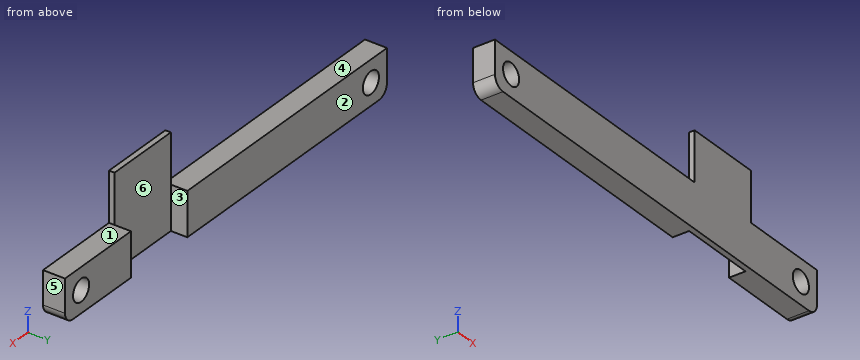
from build123d import *

# Parameters (mm, degrees)
EXTRUDE_1_DEPTH     = 12
CUT_EXTRUDE_1_DEPTH = 12
SKETCH_3_R          = 2
CUT_EXTRUDE_2_DEPTH = 12
CUT_EXTRUDE_3_DEPTH = 1
SKETCH_5_W          = 80
SKETCH_5_H          = 4
CUT_EXTRUDE_4_DEPTH = 20
EXTRUDE_2_DEPTH     = 1
SKETCH_7_W          = 0.2
SKETCH_7_H          = 8
CUT_EXTRUDE_5_DEPTH = 1
SKETCH_8_R          = 2
EXTRUDE_3_DEPTH     = 4
SKETCH_9_W          = 80
SKETCH_9_H          = 8
CUT_EXTRUDE_6_DEPTH = 10
SKETCH_10_W         = 14
SKETCH_10_H         = 8
CUT_EXTRUDE_7_DEPTH = 2
SKETCH_11_W         = 14
SKETCH_11_H         = 9
EXTRUDE_4_DEPTH     = 2
SKETCH_12_W         = 14
SKETCH_12_H         = 1
CUT_EXTRUDE_8_DEPTH = 20


with BuildPart() as part:
    # 草图1 → 凸台-拉伸1 (new body)
    with BuildSketch(Plane(origin=(0, 0, 0), x_dir=(1, 0, 0), z_dir=(0, 1, 0))):
        Polygon((-40, -6), (0, -6), (40, -6), (40, 0), (40, 6), (0, 6), (-36, 6), (-40, 6), align=None)
    extrude(amount=EXTRUDE_1_DEPTH)

    # 草图2 → 切除-拉伸1 (cut)
    with BuildSketch(Plane.XY.offset(6)):
        Polygon((-28, 0), (0, 0), (28, 0), (28, 4), (28, 8), (-28, 8), (-28, 4), align=None)
        Polygon((-40, 4), (-32, 4), (-32, 8), (-32, 12), (-40, 12), align=None)
        Polygon((32, 8), (32, 4), (40, 4), (40, 12), (32, 12), align=None)
    extrude(amount=-CUT_EXTRUDE_1_DEPTH, mode=Mode.SUBTRACT)

    # 草图3 → 切除-拉伸2 (cut)
    with BuildSketch(Plane(origin=(0, 12, 0), x_dir=(1, 0, 0), z_dir=(0, 1, 0))):
        with BuildLine():
            Line((-40, 6), (-40, 4))
            ThreePointArc((-40, 4), (-39.414213562, 5.414213562), (-38, 6))
            Line((-38, 6), (-40, 6))
        make_face()
        with Locations(Location((-36, 2, 0), (0, 0, 270))):
            Circle(SKETCH_3_R)
        with BuildLine():
            ThreePointArc((40, 4), (39.414213562, 5.414213562), (38, 6))
            Line((38, 6), (40, 6))
            Line((40, 6), (40, 4))
        make_face()
        with Locations(Location((36, 2, 0), (0, 0, 270))):
            Circle(SKETCH_3_R)
    extrude(amount=-CUT_EXTRUDE_2_DEPTH, mode=Mode.SUBTRACT)

    # 草图4 → 切除-拉伸3 (cut)
    with BuildSketch(Plane(origin=(0, 12, 0), x_dir=(1, 0, 0), z_dir=(0, 1, 0))):
        Polygon((-21.1, 0), (-21.1, 6), (-16.6, 6), (-12.1, 6), (12.08, 6), (16.6, 6), (21.12, 6), (21.12, -1), (21.12, -6), (16.6, -6), (12.08, -6), (12.08, -1), (12.08, 0), (-12.1, 0), (-12.1, -6), (-16.6, -6), (-21.1, -6), align=None)
    extrude(amount=-CUT_EXTRUDE_3_DEPTH, mode=Mode.SUBTRACT)

    # 草图5 → 切除-拉伸4 (cut)
    with BuildSketch(Plane(origin=(0, 12, 0), x_dir=(1, 0, 0), z_dir=(0, 1, 0))):
        with Locations((0, -4)):
            Rectangle(SKETCH_5_W, SKETCH_5_H)
    extrude(amount=-CUT_EXTRUDE_4_DEPTH, mode=Mode.SUBTRACT)

    # 草图6 → 凸台-拉伸2 (add)
    with BuildSketch(Plane(origin=(0, 12, 0), x_dir=(1, 0, 0), z_dir=(0, 1, 0))):
        Polygon((12.08, 0), (12.08, 6), (-21.1, 6), (-21.1, -2), (-12.1, -2), (-12.1, 0), align=None)
    extrude(amount=-EXTRUDE_2_DEPTH)

    # 草图7 → 切除-拉伸5 (cut)
    with BuildSketch(Plane(origin=(0, 12, 0), x_dir=(1, 0, 0), z_dir=(0, 1, 0))):
        with Locations((21.22, 2)):
            Rectangle(SKETCH_7_W, SKETCH_7_H)
        with Locations((11.98, 2)):
            Rectangle(SKETCH_7_W, SKETCH_7_H)
    extrude(amount=-CUT_EXTRUDE_5_DEPTH, mode=Mode.SUBTRACT)

    # 草图8 → 凸台-拉伸3 (add)
    # profile 1 of 2: a face of its own
    with BuildSketch(Plane(origin=(0, 12, 0), x_dir=(1, 0, 0), z_dir=(0, 1, 0))):
        with BuildLine():
            Line((-32, -2), (-40, -2))
            Line((-40, -2), (-40, 4))
            ThreePointArc((-40, 4), (-39.414213562, 5.414213562), (-38, 6))
            Line((-38, 6), (-32, 6))
            Line((-32, 6), (-32, -2))
        make_face()
        with Locations(Location((-36, 2, 0), (0, 0, 270))):
            Circle(SKETCH_8_R, mode=Mode.SUBTRACT)
    # profile 2 of 2: a face of its own
    with BuildSketch(Plane(origin=(0, 12, 0), x_dir=(1, 0, 0), z_dir=(0, 1, 0))):
        with BuildLine():
            Line((32, -2), (32, 6))
            Line((32, 6), (38, 6))
            ThreePointArc((38, 6), (39.414213562, 5.414213562), (40, 4))
            Line((40, 4), (40, -2))
            Line((40, -2), (32, -2))
        make_face()
        with Locations(Location((36, 2, 0), (0, 0, 270))):
            Circle(SKETCH_8_R, mode=Mode.SUBTRACT)
    extrude(amount=-EXTRUDE_3_DEPTH)

    # 草图9 → 切除-拉伸6 (cut)
    with BuildSketch(Plane.XY.offset(2)):
        with Locations((0, 4)):
            Rectangle(SKETCH_9_W, SKETCH_9_H)
    extrude(amount=-CUT_EXTRUDE_6_DEPTH, mode=Mode.SUBTRACT)

    # 草图10 → 切除-拉伸7 (cut)
    with BuildSketch(Plane(origin=(0, 12, 0), x_dir=(1, 0, 0), z_dir=(0, 1, 0))):
        with Locations((16.6, 2)):
            Rectangle(SKETCH_10_W, SKETCH_10_H)
    extrude(amount=-CUT_EXTRUDE_7_DEPTH, mode=Mode.SUBTRACT)

    # 草图11 → 凸台-拉伸4 (add)
    with BuildSketch(Plane(origin=(0, 10, 0), x_dir=(1, 0, 0), z_dir=(0, 1, 0))):
        with Locations((16.6, -6.5)):
            Rectangle(SKETCH_11_W, SKETCH_11_H)
    extrude(amount=-EXTRUDE_4_DEPTH)

    # 草图12 → 切除-拉伸8 (cut)
    with BuildSketch(Plane(origin=(0, 0, -6), x_dir=(-1, 0, 0), z_dir=(0, 0, -1))):
        with Locations((-16.6, 9.5)):
            Rectangle(SKETCH_12_W, SKETCH_12_H)
    extrude(amount=-CUT_EXTRUDE_8_DEPTH, mode=Mode.SUBTRACT)


solid = part.part
For this review, take the finished solid that the model builds, in its own axes (mm). Face numbers are marked on the shaded views. A direction names the side the tool comes from. Give positions to 0.01 mm unless a question says otherwise; leave off trailing zeros. Loops run counter-clockwise (first coordinate to the right, second up) from the corner with the lowest first, then second, coordinate; pieces in that order, holes last.
Item 1: Draft analysis for pull direction X (two halves, no side actions). For the marked faces 4, 5 and 6, state which applies: +X half, -X half, draft (parallel to the pull), parting line (faces both ways), or undercut.
Item 2: Tool access review of the marked faces 1, 2 and 3: name each direction out of +Z, -Z, +X, -X, +Y, -Y from which nothing blocks a thin tool from reaching the whole face with its end or side.
Item 3: Take a section at C-C, the plane z = 1.25. State the section outline as (x, y) points.
Item 4: Take a section at A-A, the plane x = 36. State the section outline as (y, z) points.
Item 5: For line 1 along X through (y, z) = (11.15, 0.25); line 2 along Z through (x, y) = (-3, 11.45); line 3 along Z through (x, y) = (37, 10.85), list the stretches that pass through material, from the lowest coordinate up.
Item 6: Insertion check: pin 1 (1.1 mm diameter, centred on y = 8.5, z = 7.5, fed in from -X); pin 2 (2 mm diameter, centred on x = -8.5, y = 10, fed in from +Z); pin 3 (1.1 mm diameter, centred on y = 8.5, z = 8, fed in from +X). Each pin has a flat end and moves straight along its axis. Give the tip position at first contact, or say it passes through.
Item 7: Take a section at D-D, the plane x = 8. State the section outline as (y, z) points.
Item 8: Take a section at B-B, the plane z = -2. State the section outline as (x, y) points.
Calculated:
1. face 4: draft
1. face 5: +X half
1. face 6: undercut
2. face 1: +Z, +X, +Y, -Y
2. face 2: +Z, -Z, +X, -X, +Y
2. face 3: +Z, -Z, +Y
3. outline: (-40, 8) - (40, 8) - (40, 12) - (23.6, 12) - (23.6, 9) - (9.6, 9) - (9.6, 12) - (-40, 12) - close
4. outline: (8, -6) - (12, -6) - (12, -4) - (8, -4) - close; (8, 0) - (12, 0) - (12, 2) - (8, 2) - close
5. line 1: x = -40 to 9.6, 23.6 to 40
5. line 2: z = -6 to 2
5. line 3: z = -6 to -3.73, -0.27 to 2
6. pin 1: stops at x = 9.6
6. pin 2: stops at z = 2
6. pin 3: stops at x = 23.6
7. outline: (8, -6) - (12, -6) - (12, 2) - (8, 2) - close
8. outline: (-40, 8) - (-38, 8) - (-38, 12) - (-40, 12) - close; (-34, 8) - (34, 8) - (34, 12) - (23.6, 12) - (23.6, 9) - (9.6, 9) - (9.6, 12) - (-34, 12) - close; (38, 8) - (40, 8) - (40, 12) - (38, 12) - close
